Check sheet for the modelled part. Datum: model origin and axes. Units: mm. A direction names the side the tool comes from. Coordinates: 2 decimals unless noted, no trailing zeros. Loops run counter-clockwise (first coordinate to the right, second up) from the corner with the lowest first, then second, coordinate; pieces in that order, holes last. Notation, with made-up numbers: M 47,38 L 59,38 A21 cw 59,44 Z; hole C -39.75,-20 d5. An arc over 180 degrees is marked long. Write each question's results on one line, items separated by ' | '. Start each with the question number.
from build123d import *

# Parameters (mm, degrees)
F0_W     = 78.413494
F0_H     = 93.491562
F0_W_2   = 42.211123
F0_H_2   = 30.062646
F1_DEPTH = 25.4
F3_DEPTH = 25.4


with BuildPart() as f1:
    # F0 (on Top) → F1 (new body)
    with BuildSketch(Plane.XY):
        with Locations((-4.330378, 2.591286)):
            Rectangle(F0_W, F0_H)
        with Locations((-1.256664, -15.031323)):
            Rectangle(F0_W_2, F0_H_2, mode=Mode.SUBTRACT)
    extrude(amount=F1_DEPTH)

    # F2 (on face) → F3 (join)
    with BuildSketch(Plane.YZ.offset(34.876369)):
        Polygon((49.337067, 0), (49.337067, 12.7), (-44.154495, 25.4), (-44.154495, 0), align=None)
        Polygon((-44.154495, 25.4), (49.337067, 12.7), (49.337067, 25.4), align=None)
    extrude(amount=F3_DEPTH)


solid = f1.part
Item 1: Thickness scan on line 1 (Y direction, x = 17, z = 17.75); line 2 (X direction, y = -26.5, z = 7.5). Record the ranges inside material, lowest first.
Item 2: Release check for a two-part mould opening along X. For faces 1 (the face through (8, -44.154, 13)), 2 (the face through (-43.537, 2, 13)), 3 (the face through (-22.362, -15, 13)) record: +X half, -X half, draft (parallel to the pull), parting line (faces both ways), or undercut.
Item 3: Section check A-A (x = -21). Record the cut outline in (y, z).
Item 4: Tool access check on faces 4 (the face through (-2, -30.063, 13)), 5 (the face through (8, 49.337, 13)). Record the directions out of +Z, -Z, +X, -X, +Y, -Y that give a thin tool (end or side, any length) a straight path to the whole face; none if there is none.
Item 5: Section check C-C (z = 9.75). Record the cut outline in (x, y), plus the area to 3 significant figures.
Item 6: Section check B-B (y = -24.5). Record the cut outline in (x, z).
Computed values:
1) line 1: y = -44.15 to -30.06, 0 to 49.34 | line 2: x = -43.54 to -22.36, 19.85 to 60.28
2) face 1: draft | face 2: -X half | face 3: undercut
3) outline: M -44.15,0 L -30.06,0 L -30.06,25.4 L -44.15,25.4 Z; M 0,0 L 49.34,0 L 49.34,25.4 L 0,25.4 Z
4) face 4: +Z, -Z | face 5: +Z, -Z, +X, -X, +Y
5) outline: M -43.54,-44.15 L 60.28,-44.15 L 60.28,49.34 L -43.54,49.34 Z; hole M -22.36,-30.06 L 19.85,-30.06 L 19.85,0 L -22.36,0 Z | area: 8,440 mm²
6) outline: M -43.54,0 L -22.36,0 L -22.36,25.4 L -43.54,25.4 Z; M 19.85,0 L 60.28,0 L 60.28,25.4 L 19.85,25.4 Z
